```python
from build123d import *

# Parameters (mm, degrees)
F1_DEPTH = 10
F2_R     = 2
F3_R     = 2.3474
F4_DEPTH = 25


with BuildPart() as f1:
    # F0 (on Top) → F1 (new body)
    with BuildSketch(Plane.XY):
        Polygon((0, 40), (0, 0), (30, 0), (30, 10), (10, 10), (10, 40), align=None)
    extrude(amount=F1_DEPTH)

    # F2
    f2_edges = [f1.edges().sort_by_distance(p)[0] for p in [
        (0, 20, 10),
        (15, 0, 10),
        (30, 5, 10),
        (20, 10, 10),
        (10, 25, 10),
        (5, 40, 10),
        (0, 20, 0),
        (15, 0, 0),
        (30, 5, 0),
        (20, 10, 0),
        (10, 25, 0),
        (5, 40, 0),
        (10, 40, 5),
        (0, 40, 5),
        (10, 10, 5),
        (30, 10, 5),
        (0, 0, 5),
        (30, 0, 5),
    ]]
    fillet(f2_edges, radius=F2_R)

    # F3 (on face) → F4 (cut)
    with BuildSketch(Plane.XY.offset(10)):
        with Locations((6.827323, 4.902695)):
            Circle(F3_R)
    extrude(amount=-F4_DEPTH, mode=Mode.SUBTRACT)


solid = f1.part
```
Design review of the part built by this model. Coordinates are the model's own, in mm. A direction names the side the tool comes from. Give positions to 0.01 mm unless a question says otherwise; leave off trailing zeros. Order: outer loops, then holes, each group sorted by start corner. A loop starts at its lowest first (then second) coordinate and runs counter-clockwise, first axis right, second up. Notation, with made-up numbers: (-3, 34.25) -> (29, 34.25) arc R24 cw to (29, 60.25) -> close; hole circle Ø10 at (-38.75, 1.25). An arc over 180 degrees is marked (long way). Write item = value, one per line. Start each with the question number.
(1) We need section A-A on x = 19.25. Write out the cut boundary in (y, z), plus the area to 3 significant figures.
(2) We need section B-B on z = 5.5. Write out the cut boundary in (x, y), plus the area to 3 significant figures.
(3) For faces 1 (the face through (10, 25, 5)), 2 (the face through (9.43, 25.18, 0.6)), 3 (the face through (19.89, 9.43, 9.4)), list the 3-axis set-ups (+Z, -Z, +X, -X, +Y, -Y) from which the entire face can be reached by the end or side of a thin tool; tool diameter is ignored.
(4) To check wall thickness, follow line 1 along Y through (x, z) = (18.5, 5.75); line 2 along Y through (x, z) = (8, 7). State the ranges of each line that lie inside material, in increasing order.
(5) For pin 1 (1.5 mm diameter, centred on x = 17.5, y = 12, fed in from +Z); pin 2 (1.5 mm diameter, centred on y = 18, z = 1, fed in from -X); pin 3 (1 mm diameter, centred on x = 24, z = 3, fed in from +Y), all flat-tipped, find the tip position at first contact; note any pin that passes through.
(6) We need section D-D on x = 6.75. Write out the cut boundary in (y, z).
Numbers:
q1.outline = (0, 2) arc R2 ccw to (2, 0) -> (8, 0) arc R2 ccw to (10, 2) -> (10, 8) arc R2 ccw to (8, 10) -> (2, 10) arc R2 ccw to (0, 8) -> close
q1.area = 96.6 mm^2
q2.outline = (0, 2) arc R2 ccw to (2, 0) -> (28, 0) arc R2 ccw to (30, 2) -> (30, 8) arc R2 ccw to (28, 10) -> (12, 10) arc R2 cw to (10, 12) -> (10, 38) arc R2 ccw to (8, 40) -> (2, 40) arc R2 ccw to (0, 38) -> close; hole circle Ø4.69 at (6.83, 4.9)
q2.area = 579 mm^2
q3.face_1 = +Z, -Z, +X, +Y
q3.face_2 = -Z, +X, +Y
q3.face_3 = +Z, +X, +Y
q4.line_1 = 0 to 10
q4.line_2 = 0 to 2.87, 6.94 to 40
q5.pin_1 = through
q5.pin_2 = 0.02
q5.pin_3 = 10
q6.outline = (0, 2) arc R2 ccw to (2, 0) -> (2.56, 0) -> (2.56, 10) -> (2, 10) arc R2 ccw to (0, 8) -> close; (7.25, 0) -> (38, 0) arc R2 ccw to (40, 2) -> (40, 8) arc R2 ccw to (38, 10) -> (7.25, 10) -> close
